Here's the drawing with two shaded views (mm, measured from the low corner). I have some questions. A direction names the side the tool comes from. Give positions to 0.01 mm unless a question says otherwise; leave off trailing zeros. Write each loop counter-clockwise with the first axis right and the second up, starting at its lowest first coordinate (ties: lowest second). Pieces come first, ordered by that corner, then holes. Notation, with made-up numbers: M 52,16 L 85,16 A29 cw 85,41 Z; hole C -28.75,49 d6. An arc over 180 degrees is marked long. Answer as a JSON object with one key per item and string values. Group by question number.
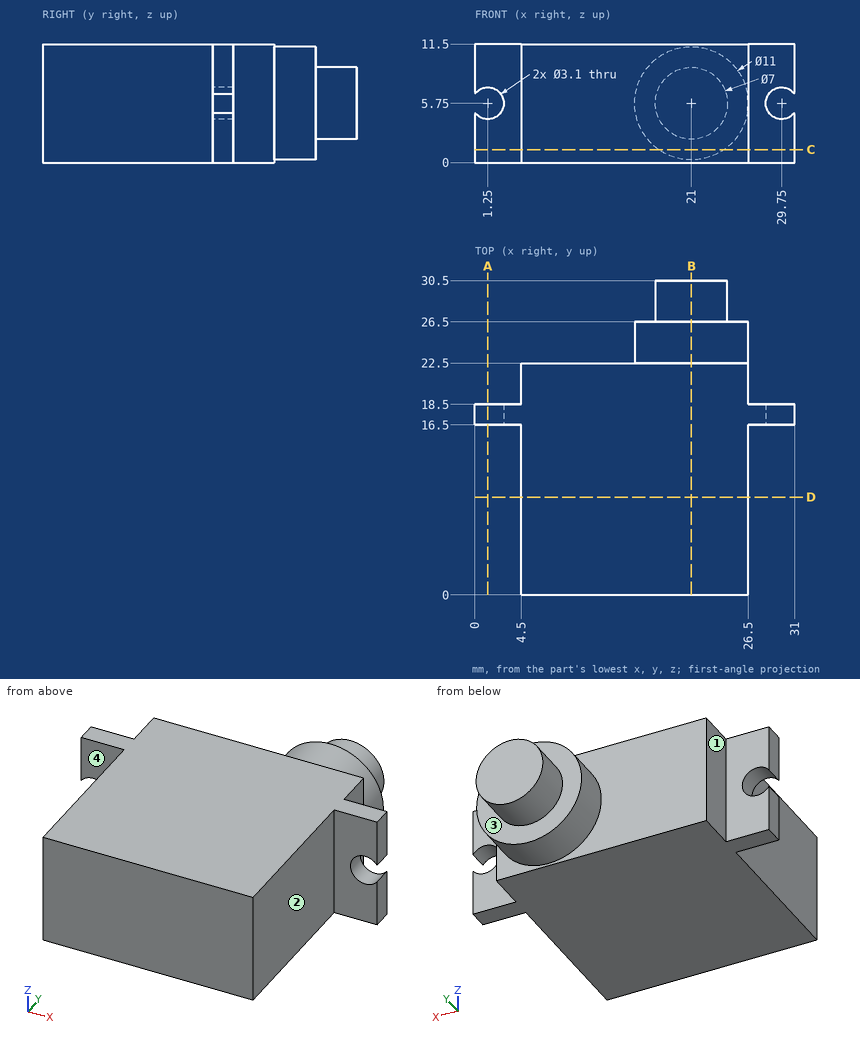
1) For the marked faces 1, 2, 3 and 4, which set-ups out of +Z, -Z, +X, -X, +Y, -Y let a thin tool reach every point of the face, with its end or its side?
2) Please list where these lines run through material, in increasing order: line 1 along Z through (x, y) = (1.25, 17.75); line 2 along Y through (x, z) = (11.5, 8); line 3 along Z through (x, y) = (28.5, 18). Write a range as from..to.
3) I'm going to push flat-ended pins straight in: pin 1 (4 mm diameter, centred on x = 1.25, z = 5.75, fed in from +Y); pin 2 (1.2 mm diameter, centred on y = 20, z = 7.5, fed in from +X); pin 3 (5 mm diameter, centred on y = 13.5, z = 5, fed in from -X). Where does each tip first touch, or does it pass through?
4) If we section it at C-C, the plane z = 1.25: List the corners of the cut face in (x, y) for me, plus the area to 3 significant figures.
5) If we section it at A-A, the plane x = 1.25: List the corners of the cut face in (y, z) for me.
6) If we section it at D-D, the plane y = 9.5: List the corners of the cut face in (x, z) for me.
7) If we section it at B-B, the plane x = 21: List the corners of the cut face in (y, z) for me.
Taken from the geometry:
{
 "1": {"face 1": "+Z, -Z, -X, +Y", "face 2": "+Z, -Z, +X, -Y", "face 3": "+Y", "face 4": "+Z, -Z, -X, -Y"},
 "2": {"line 1": "0..4.2, 7.3..11.5", "line 2": "0..22.5", "line 3": "0..4.83, 6.67..11.5"},
 "3": {"pin 1": "y = 18.5", "pin 2": "x = 26.5", "pin 3": "x = 4.5"},
 "4": {"outline": "M 0,16.5 L 4.5,16.5 L 4.5,0 L 26.5,0 L 26.5,16.5 L 31,16.5 L 31,18.5 L 26.5,18.5 L 26.5,22.5 L 24.16,22.5 L 24.16,26.5 L 17.84,26.5 L 17.84,22.5 L 4.5,22.5 L 4.5,18.5 L 0,18.5 Z", "area": "538 mm²"},
 "5": {"outline": "M 16.5,0 L 18.5,0 L 18.5,4.2 L 16.5,4.2 Z; M 16.5,7.3 L 18.5,7.3 L 18.5,11.5 L 16.5,11.5 Z"},
 "6": {"outline": "M 4.5,0 L 26.5,0 L 26.5,11.5 L 4.5,11.5 Z"},
 "7": {"outline": "M 0,0 L 22.5,0 L 22.5,0.25 L 26.5,0.25 L 26.5,2.25 L 30.5,2.25 L 30.5,9.25 L 26.5,9.25 L 26.5,11.25 L 22.5,11.25 L 22.5,11.5 L 0,11.5 Z"}
}
